Input: part model. Units: mm. Frame: model coordinates. Face numbers are marked on the shaded views. A direction names the side the tool comes from. Give positions to 0.01 mm unless a question says otherwise; leave off trailing zeros. Order: outer loops, then holes, each group sorted by start corner. A loop starts at its lowest first (then second) coordinate and runs counter-clockwise, first axis right, second up. Notation, with made-up numbers: (-2.75, 7.25) - (33.25, 7.25) arc R31 cw to (33.25, 43.25) - close; hole circle Ø11 at (37.25, 67.5). An arc over 180 degrees is marked (long way). Answer in a Markdown table with one row per item. Add a question column.
from build123d import *

# Parameters (mm, degrees)
F0_W     = 50
F0_H     = 20
F1_DEPTH = 6
F2_W     = 6
F2_H     = 20
F3_DEPTH = 20
F4_R     = 3.5
F5_DEPTH = 25
F6_SIZE  = 5
F7_R     = 3
F8_DEPTH = 25


# Not quite as in the source:
# - a pattern or mirror of a feature is missing from the dataset's text; its kind, count and spacing are read off the source's solid


with BuildPart() as f1:
    # F0 (on Top) → F1 (new body)
    with BuildSketch(Plane.XY):
        Rectangle(F0_W, F0_H)
    extrude(amount=F1_DEPTH)

    # F2 (on face) → F3 (join)
    with BuildSketch(Plane.XY.offset(6)):
        with Locations((-6.5, 0)):
            Rectangle(F2_W, F2_H)
    f3 = extrude(amount=F3_DEPTH)

    # F3_copies: F3 across plane
    add(f3.mirror(Plane(origin=(0, 0, 0), x_dir=(0, 0, 1), z_dir=(1, 0, 0))))

    # F4 (on face) → F5 (cut)
    with BuildSketch(Plane.YZ.offset(-3.5)):
        with Locations((0, 18)):
            Circle(F4_R)
    f5 = extrude(amount=-F5_DEPTH, mode=Mode.SUBTRACT)

    # F5_copies: F5 across plane
    add(f5.mirror(Plane(origin=(0, 0, 0), x_dir=(0, 0, 1), z_dir=(1, 0, 0))), mode=Mode.SUBTRACT)

    # F6
    f6_edges = [f1.edges().sort_by_distance(p)[0] for p in [
        (-6.5, -10, 26),
        (-6.5, 10, 26),
        (6.5, -10, 26),
        (6.5, 10, 26),
    ]]
    chamfer(f6_edges, length=F6_SIZE)

    # F7 (on face) → F8 (cut)
    with BuildSketch(Plane.XY.offset(6)):
        with Locations((-17.25, 0)):
            Circle(F7_R)
    f8 = extrude(amount=-F8_DEPTH, mode=Mode.SUBTRACT)

    # F8_copies: F8 across plane
    add(f8.mirror(Plane(origin=(0, 0, 0), x_dir=(0, 0, 1), z_dir=(1, 0, 0))), mode=Mode.SUBTRACT)


solid = f1.part
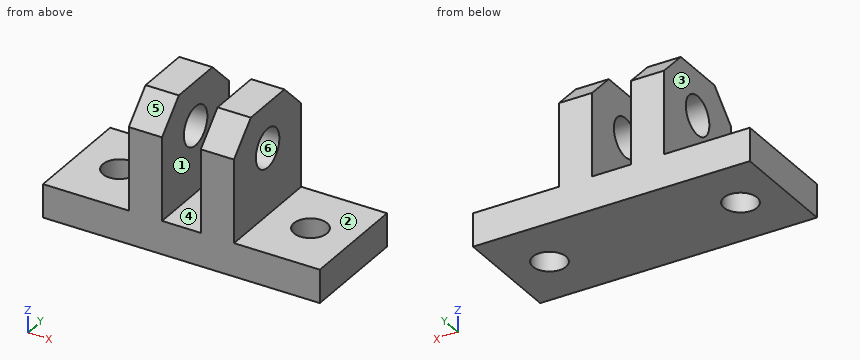
Q1. Section B-B, the plane z = 18. Return loops of the section in (x, y).
Q2. Pull-direction query (Y, two-part tool) for the marked faces 4, 5 and 6; classes: +Y half, -Y half, draft (parallel to the pull), parting line (faces both ways), or undercut.
Q3. Contact query for flat-ended pins moving along their axis: P1, Ø2, axis at y = -3, z = 19.5, coming from the -X side; P2, Ø4, axis at x = 19.5, y = 4.5, coming from the +Z side; P3, Ø11, axis at y = 0, z = 18, coming from the +X side. Output: stop coordinate, or through.
Q4. Section A-A, the plane x = -17.25. Return loops of the section in (y, z), then the cut area to 3 significant figures.
Q5. Line query: probe 1 along Y at (x, z) = (17.25, 2.1); probe 2 along X at (y, z) = (-7, 12.75); probe 3 along X at (y, z) = (-1.75, 4). Output: solid intervals per line, ascending.
Q6. Section C-C, the plane y = 0. Return loops of the section in (x, z).
Q7. Access query for the marked faces 1, 2 and 3. Directions: +Z, -Z, +X, -X, +Y, -Y. A direction counts if a zero-diameter tool reaches every point of the face in a straight line with its end or side. Return the directions, or none.
Q8. Section D-D, the plane z = 22.75. Return loops of the section in (x, y).
Computed:
| question | item | result |
|---|---|---|
| 1 | outline | (-9.5, -10) - (-3.5, -10) - (-3.5, -3.5) - (-9.5, -3.5) - close; (-9.5, 3.5) - (-3.5, 3.5) - (-3.5, 10) - (-9.5, 10) - close; (3.5, -10) - (9.5, -10) - (9.5, -3.5) - (3.5, -3.5) - close; (3.5, 3.5) - (9.5, 3.5) - (9.5, 10) - (3.5, 10) - close |
| 2 | face 4 | draft |
| 2 | face 5 | -Y half |
| 2 | face 6 | undercut |
| 3 | P1 | stops at x = -9.5 |
| 3 | P2 | stops at z = 6 |
| 3 | P3 | stops at x = 9.5 |
| 4 | outline | (-10, 0) - (-3, 0) - (-3, 6) - (-10, 6) - close; (3, 0) - (10, 0) - (10, 6) - (3, 6) - close |
| 4 | area | 84.0 mm^2 |
| 5 | probe 1 | y = -10 to -3, 3 to 10 |
| 5 | probe 2 | x = -9.5 to -3.5, 3.5 to 9.5 |
| 5 | probe 3 | x = -25 to -19.69, -14.81 to 14.81, 19.69 to 25 |
| 6 | outline | (-25, 0) - (-20.25, 0) - (-20.25, 6) - (-25, 6) - close; (-14.25, 0) - (14.25, 0) - (14.25, 6) - (9.5, 6) - (9.5, 14.5) - (3.5, 14.5) - (3.5, 6) - (-3.5, 6) - (-3.5, 14.5) - (-9.5, 14.5) - (-9.5, 6) - (-14.25, 6) - close; (-9.5, 21.5) - (-3.5, 21.5) - (-3.5, 26) - (-9.5, 26) - close; (3.5, 21.5) - (9.5, 21.5) - (9.5, 26) - (3.5, 26) - close; (20.25, 0) - (25, 0) - (25, 6) - (20.25, 6) - close |
| 7 | face 1 | +Z, +Y, -Y |
| 7 | face 2 | +Z, +X, +Y, -Y |
| 7 | face 3 | +Z, -X, +Y, -Y |
| 8 | outline | (-9.5, -8.25) - (-3.5, -8.25) - (-3.5, 8.25) - (-9.5, 8.25) - close; (3.5, -8.25) - (9.5, -8.25) - (9.5, 8.25) - (3.5, 8.25) - close |
